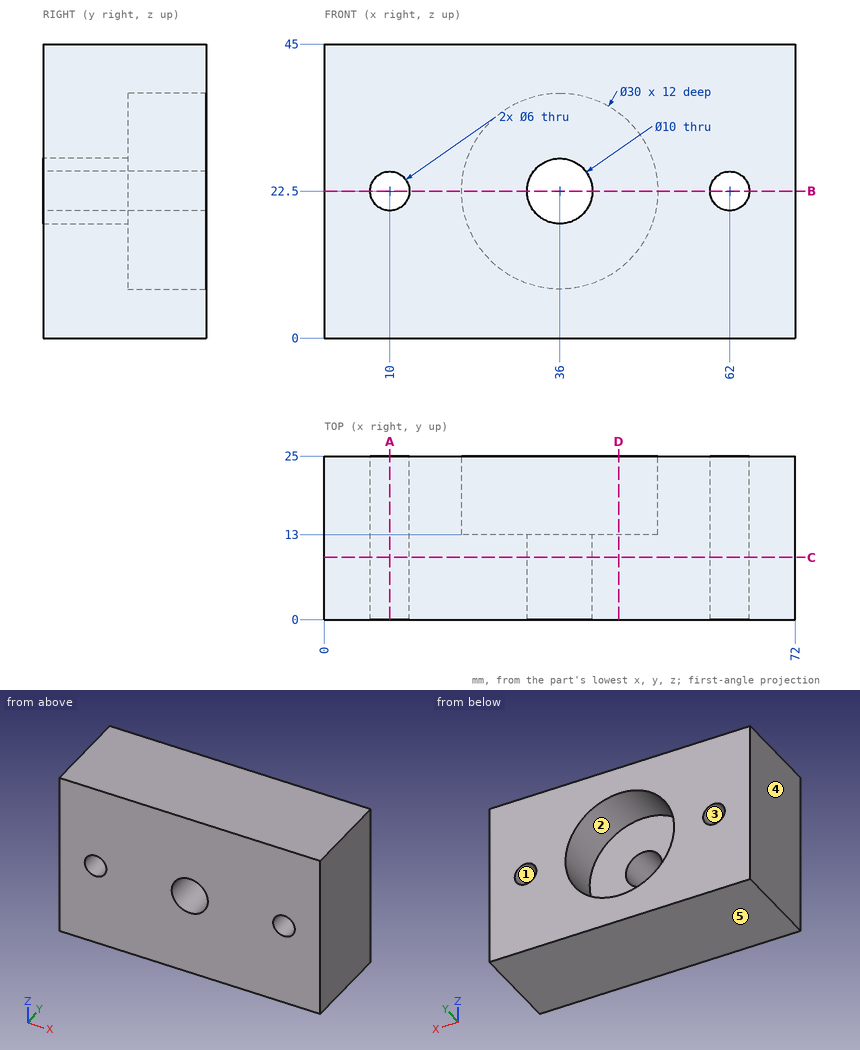
Job drawing, mm, ordinate dimensions from the low corner. One solid piece. A direction names the side the tool comes from. Coordinates: 2 decimals unless noted, no trailing zeros. Order: outer loops, then holes, each group sorted by start corner. A loop starts at its lowest first (then second) coordinate and runs counter-clockwise, first axis right, second up. Notation, with made-up numbers: (-22, -9) - (12, -9) arc R13 ccw to (12, 0) - close; hole circle Ø9 at (86, 57). An arc over 180 degrees is marked (long way). Return JSON: item names as keys, results as strings. Group by question number.
1) Saw through at C-C, the plane y = 9.5. Write the cut outline in (x, z).
2) Tool access for the marked faces 1 and 2: list every direction of +Z, -Z, +X, -X, +Y, -Y with a clear straight run to the whole face (end or side of a thin tool).
3) Flat gauge pins, fed straight in: P1, Ø12, axis at x = 55.5, y = 15.5, coming from the -Z side; P2, Ø11.5, axis at x = 36, z = 22.5, coming from the +Y side. Where does each tip first touch, or does it go through?
4) Probe line 1 (X direction, y = 18.5, z = 22.5); line 2 (X direction, y = 8, z = 22.5); line 3 (Y direction, x = 47, z = 23.5). List the from-to ranges inside material, lowest first. Write a range as from..to.
5) Mould opens along X. For the marked faces 3, 4 and 5 say: released by +X, released by -X, zero draft, split by the parting line, or undercut.
6) Saw through at B-B, the plane z = 22.5. Write the cut outline in (x, y), plus the area to 3 significant figures.
7) Saw through at D-D, the plane x = 45. Write the cut outline in (y, z), plus the area to 3 significant figures.
8) Saw through at A-A, the plane x = 10. Write the cut outline in (y, z), plus the area to 3 significant figures.
Values found:
{
 "1": {"outline": "(0, 0) - (72, 0) - (72, 45) - (0, 45) - close; hole circle Ø6 at (10, 22.5); hole circle Ø10 at (36, 22.5); hole circle Ø6 at (62, 22.5)"},
 "2": {"face 1": "+Y, -Y", "face 2": "+Y"},
 "3": {"P1": "stops at z = 0", "P2": "stops at y = 13"},
 "4": {"line 1": "x = 0..7, 13..21, 51..59, 65..72", "line 2": "x = 0..7, 13..31, 41..59, 65..72", "line 3": "y = 0..13"},
 "5": {"face 3": "undercut", "face 4": "released by -X", "face 5": "zero draft"},
 "6": {"outline": "(0, 0) - (7, 0) - (7, 25) - (0, 25) - close; (13, 0) - (31, 0) - (31, 13) - (21, 13) - (21, 25) - (13, 25) - close; (41, 0) - (59, 0) - (59, 25) - (51, 25) - (51, 13) - (41, 13) - close; (65, 0) - (72, 0) - (72, 25) - (65, 25) - close", "area": "1,010 mm²"},
 "7": {"outline": "(0, 0) - (25, 0) - (25, 10.5) - (13, 10.5) - (13, 34.5) - (25, 34.5) - (25, 45) - (0, 45) - close", "area": "837 mm²"},
 "8": {"outline": "(0, 0) - (25, 0) - (25, 19.5) - (0, 19.5) - close; (0, 25.5) - (25, 25.5) - (25, 45) - (0, 45) - close", "area": "975 mm²"}
}
